```python
from build123d import *

# Parameters (mm, degrees)
F1_DEPTH = 25.4
F3_DEPTH = 38.1


with BuildPart() as f1:
    # F0 (on Top) → F1 (new body)
    with BuildSketch(Plane.XY):
        with BuildLine():
            ThreePointArc((146.05, 70.1765862209), (127, 89.2265862209), (107.95, 70.1765862209))
            Line((107.95, 70.1765862209), (146.05, 70.1765862209))
        make_face()
        with BuildLine():
            Line((146.05, 70.1765862209), (107.95, 70.1765862209))
            ThreePointArc((107.95, 70.1765862209), (127, 51.1265862209), (146.05, 70.1765862209))
        make_face()
        with BuildLine():
            Line((25.4, 70.1765862209), (0, 50.8))
            Line((0, 50.8), (0, 0))
            Line((0, 0), (254, 0))
            Line((254, 0), (254, 50.8))
            Line((254, 50.8), (228.6, 70.1765862209))
            Line((228.6, 70.1765862209), (146.05, 70.1765862209))
            ThreePointArc((146.05, 70.1765862209), (127, 51.1265862209), (107.95, 70.1765862209))
            Line((107.95, 70.1765862209), (25.4, 70.1765862209))
        make_face()
    extrude(amount=F1_DEPTH)

    # F2 (on face) + F0 (on Top) → F3 (join)
    with BuildSketch(Plane.XY):
        with BuildLine():
            ThreePointArc((107.95, 70.1765862209), (127, 51.1265862209), (146.05, 70.1765862209))
            Line((146.05, 70.1765862209), (107.95, 70.1765862209))
        make_face()
    with BuildSketch(Plane.XY):
        with BuildLine():
            ThreePointArc((146.05, 70.1765862209), (127, 89.2265862209), (107.95, 70.1765862209))
            Line((107.95, 70.1765862209), (146.05, 70.1765862209))
        make_face()
    extrude(amount=F3_DEPTH)


solid = f1.part
```
Work out the finished part from the listing and answer in its coordinate system (mm). A direction names the side the tool comes from. Give positions to 0.01 mm unless a question says otherwise; leave off trailing zeros. Order: outer loops, then holes, each group sorted by start corner. A loop starts at its lowest first (then second) coordinate and runs counter-clockwise, first axis right, second up. Notation, with made-up numbers: M -28,30 L -16,30 A8 cw -16,34 Z; hole C -3,19 d8. An arc over 180 degrees is marked long. Return JSON: item names as keys, results as strings.
1) Section D-D, the plane y = 8.5 is taken. Write down the section's boundary in (x, z), plus the area to 3 significant figures.
Resolved:
{"outline": "M 0,0 L 254,0 L 254,25.4 L 0,25.4 Z", "area": "6,450 mm^2"}
2) Straight lines are drawn through the part: line 1 along Z through (x, y) = (207, 55); line 2 along Y through (x, z) = (41, 9); line 3 along X through (y, z) = (61.5, 22.5). For each, find the intervals that lie inside material, in ascending order. Write a range as [from, to].
Resolved:
{"line 1": "[0, 25.4]", "line 2": "[0, 70.18]", "line 3": "[14.03, 239.97]"}
3) Section A-A, the plane z = 18 is taken. Write down the section's boundary in (x, y).
Resolved:
{"outline": "M 0,0 L 254,0 L 254,50.8 L 228.6,70.18 L 146.05,70.18 A19.05 ccw 107.95,70.18 L 25.4,70.18 L 0,50.8 Z"}
4) Section C-C, the plane y = 55.5 is taken. Write down the section's boundary in (x, z).
Resolved:
{"outline": "M 6.16,0 L 247.84,0 L 247.84,25.4 L 139.14,25.4 L 139.14,38.1 L 114.86,38.1 L 114.86,25.4 L 6.16,25.4 Z"}
5) A tool of negligible diameter and unlimited length cuts with its end or side. For faces 1 (the flat face through (188, 70.177, 13)), 2 (the flat face through (0, 26, 13)), 3 (the flat face through (67, 70.177, 13)), from which of +Z, -Z, +X, -X, +Y, -Y can it reach the whole face along a straight path? Write none if from no direction.
Resolved:
{"face 1": "+Z, -Z, +X, +Y", "face 2": "+Z, -Z, -X, +Y, -Y", "face 3": "+Z, -Z, -X, +Y"}
6) Section B-B, the plane x = 127 is taken. Write down the section's boundary in (y, z).
Resolved:
{"outline": "M 0,0 L 89.23,0 L 89.23,38.1 L 51.13,38.1 L 51.13,25.4 L 0,25.4 Z"}
7) Each of these flat-tipped pins is pushed along its axis until it touches: pin 1 (3 mm diameter, centred on x = 191.5, y = 21, fed in from +Z); pin 2 (1.5 mm diameter, centred on y = 64.5, z = 26, fed in from +X); pin 3 (8 mm diameter, centred on y = 42.5, z = 29.5, fed in from +X); pin 4 (12.5 mm diameter, centred on x = 200.5, z = 10.5, fed in from +Y). Where does it stop, or does it pass through?
Resolved:
{"pin 1": "z = 25.4", "pin 2": "x = 236.63", "pin 3": "through", "pin 4": "y = 70.18"}
